The model under review builds one solid part; all positions refer to its coordinate system, in mm. A direction names the side the tool comes from. Coordinates: 2 decimals unless noted, no trailing zeros. Write each loop counter-clockwise with the first axis right and the second up, starting at its lowest first coordinate (ties: lowest second). Pieces come first, ordered by that corner, then holes. Notation, with made-up numbers: (-1.5, 70.5) - (13.5, 70.5) arc R15 cw to (13.5, 91.5) - close; hole circle Ø11 at (11.5, 68). An arc over 180 degrees is marked (long way). Put each result on its own line as item: value.
from build123d import *

# Parameters (mm, degrees)
F0_W           = 190.5
F0_H           = 35.1282
F1_DEPTH       = 12.7
F3_DEPTH       = 190.501
F5_D           = 3.4544
F5_CSINK_D     = 9.1186
F5_CSINK_ANGLE = 82
F7_D           = 6.5278
F7_DEPTH       = 16.4846
F7_TIP         = 1.9611489744


with BuildPart() as f1:
    # F0 (on Front) → F1 (new body)
    with BuildSketch(Plane.XZ):
        with Locations((95.25, 17.5641)):
            Rectangle(F0_W, F0_H)
    extrude(amount=F1_DEPTH)

    # F2 (on face) → F3 (cut, through all)
    with BuildSketch(Plane.YZ.offset(190.5)):
        Polygon((-3.81, 35.1282), (-8.89, 35.1282), (-9.4869, 27.7622), (-3.2131, 27.7622), align=None)
    extrude(amount=-F3_DEPTH, mode=Mode.SUBTRACT)

    # F5 (through all)
    with Locations(Plane.XZ.offset(12.7)):
        with Locations((9.5504, 25.8572), (85.5853, 25.8572), (155.5623, 25.8572)):
            CounterSinkHole(F5_D / 2, F5_CSINK_D / 2, counter_sink_angle=F5_CSINK_ANGLE)

    # F7
    with Locations(Plane(origin=(0, 0, 0), x_dir=(1, 0, 0), z_dir=(0, 0, -1))):
        with Locations((25.2984, 6.35), (95.25, 6.35), (165.2016, 6.35)):
            Hole(F7_D / 2, depth=F7_DEPTH)
            with Locations((0, 0, -(F7_DEPTH + F7_TIP / 2))):  # 118° drill point
                Cone(0, F7_D / 2, F7_TIP, mode=Mode.SUBTRACT)


solid = f1.part
1. For pin 1 Ø7 at (x, y) = (75.5, -7.5) entering from +Z; pin 2 Ø4 at (x, y) = (165.2, -6.35) entering from +Z; pin 3 Ø4 at (x, z) = (85.59, 25.86) entering from -Y, all flat-tipped, find the tip position at first contact; note any pin that passes through.
Determined:
pin 1: stops at z = 35.13
pin 2: stops at z = 27.76
pin 3: stops at y = -9.76
2. Consider section B-B on x = 36.5. State the section outline as (y, z) points.
Determined:
outline: (-12.7, 0) - (0, 0) - (0, 35.13) - (-3.81, 35.13) - (-3.21, 27.76) - (-9.49, 27.76) - (-8.89, 35.13) - (-12.7, 35.13) - close
3. Machinability: for faces 1 (the cylindrical face through (22.283, -5.1, 8.358)), 2 (the flat face through (94, -12.7, 18)), 3 (the flat face through (97, -6, 27.762)), which of the approach directions +Z, -Z, +X, -X, +Y, -Y give a long, thin tool a straight path to every point of the face, cutting with its end or side? Answer none if there is none.
Determined:
face 1: -Z
face 2: +Z, -Z, +X, -X, -Y
face 3: +X, -X
4. The part is to be moulded in two halves that separate along X. For faces 4 (the cylindrical face through (83.94, -4.65, 26.38)), 5 (the flat face through (0, -6, 17)), 6 (the flat face through (94, -2, 35.128)), say which applies: +X half, -X half, draft (parallel to the pull), parting line (faces both ways), or undercut.
Determined:
face 4: undercut
face 5: -X half
face 6: draft
5. Consider section A-A on z = 4. State the section outline as (x, y) points.
Determined:
outline: (0, -12.7) - (190.5, -12.7) - (190.5, 0) - (0, 0) - close; hole circle Ø6.53 at (25.3, -6.35); hole circle Ø6.53 at (95.25, -6.35); hole circle Ø6.53 at (165.2, -6.35)
6. To check wall thickness, follow probe 1 along X at (y, z) = (-0.75, 26.5); probe 2 along X at (y, z) = (-8, 12); probe 3 along Z at (x, y) = (115.5, -8). State the ranges of each line that lie inside material, in increasing order.
Determined:
probe 1: x = 0 to 7.95, 11.15 to 83.98, 87.19 to 153.96, 157.17 to 190.5
probe 2: x = 0 to 22.48, 28.11 to 92.43, 98.07 to 162.39, 168.02 to 190.5
probe 3: z = 0 to 27.76
